from build123d import *

# Parameters (mm, degrees)
F0_W     = 101.6
F0_H     = 76.2
F1_DEPTH = 76.2
F3_DEPTH = 76.201
F5_DEPTH = 50.8


with BuildPart() as f1:
    # F0 (on Front) → F1 (new body)
    with BuildSketch(Plane.XZ):
        with Locations((21.473836, 21.002229)):
            Rectangle(F0_W, F0_H)
    extrude(amount=F1_DEPTH)

    # F2 (on face) → F3 (cut, through all)
    with BuildSketch(Plane.XY.offset(59.102229)):
        with BuildLine():
            Line((72.273836, -63.5), (72.273836, -12.7))
            ThreePointArc((72.273836, -12.7), (46.873836, -38.1), (72.273836, -63.5))
        make_face()
    extrude(amount=-F3_DEPTH, mode=Mode.SUBTRACT)

    # F4 (on face) → F5 (cut)
    with BuildSketch(Plane(origin=(-29.326164, 0, 0), x_dir=(0, -1, 0), z_dir=(-1, 0, 0))):
        with BuildLine():
            Line((76.2, 59.102229), (25.4, 59.102229))
            ThreePointArc((25.4, 59.102229), (40.278976, 23.181204), (76.2, 8.302229))
            Line((76.2, 8.302229), (76.2, 59.102229))
        make_face()
    extrude(amount=-F5_DEPTH, mode=Mode.SUBTRACT)


solid = f1.part
Work out the finished part from the listing and answer in its coordinate system (mm). A direction names the side the tool comes from. Round coordinates to 2 decimals unless told otherwise and drop trailing zeros. Write each loop counter-clockwise with the first axis right and the second up, starting at its lowest first coordinate (ties: lowest second). Pieces come first, ordered by that corner, then holes. Notation, with made-up numbers: M 57.25,-17.75 L 68.25,-17.75 A32 cw 68.25,12.25 Z; hole C 40.5,29 d10. An arc over 180 degrees is marked long. Use a Markdown table: item, result.
1) Consider line 1 (Y direction, x = 53, z = 53); line 2 (X direction, y = -41.5, z = 54.5); line 3 (X direction, y = -31, z = 43). Determine where each line is inside the solid, lowest interval first. Write a range as [from, to].
Taken from the geometry:
| item | result |
|---|---|
| line 1 | y = [-76.2, -54.64], [-21.56, 0] |
| line 2 | x = [21.47, 47.1] |
| line 3 | x = [21.47, 47.89] |
2) Which of the six approach directions +Z, -Z, +X, -X, +Y, -Y give full straight-line access (tool end or side, diameter ignored) to faces 4 (the face through (72.274, -70, 20)), 5 (the face through (-4.282, -39.886, 23.578))?
Taken from the geometry:
| item | result |
|---|---|
| face 4 | +Z, -Z, +X, +Y, -Y |
| face 5 | +Z, -X, -Y |
3) Determine the mould class of faces 1 (the face through (72.274, -6, 20)), 2 (the face through (46.88, -37.54, 21.54)), 3 (the face through (21, 0, 22)) for opening direction Y: pulls with the +Y half, pulls with the -Y half, needs draft (parallel to the pull), parting line crosses it, or undercut.
Taken from the geometry:
| item | result |
|---|---|
| face 1 | needs draft |
| face 2 | undercut |
| face 3 | pulls with the +Y half |
4) The part is cut by section B-B on z = 17. Give the vertices of the cut face in (x, y).
Taken from the geometry:
| item | result |
|---|---|
| outline | M -29.33,-47.77 L 21.47,-47.77 L 21.47,-76.2 L 72.27,-76.2 L 72.27,-63.5 A25.4 cw 72.27,-12.7 L 72.27,0 L -29.33,0 Z |
5) The part is cut by section D-D on y = -38.1. Give the vertices of the cut face in (x, z).
Taken from the geometry:
| item | result |
|---|---|
| outline | M -29.33,-17.1 L 46.87,-17.1 L 46.87,59.1 L 21.47,59.1 L 21.47,25.5 L -29.33,25.5 Z |
6) The part is cut by section A-A on x = 16. Give the vertices of the cut face in (y, z).
Taken from the geometry:
| item | result |
|---|---|
| outline | M -76.2,-17.1 L 0,-17.1 L 0,59.1 L -25.4,59.1 A50.8 cw -76.2,8.3 Z |
7) Flat-ended cylindrical pins translate along their axes: pin 1 (1.5 mm diameter, centred on x = 14, z = 23, fed in from -Y) (3 decimals); pin 2 (1 mm diameter, centred on y = -40, z = 36.5, fed in from +X). Find the tip coordinate at first contact, or state that the pin passes through.
Taken from the geometry:
| item | result |
|---|---|
| pin 1 | stops at y = -41.235 |
| pin 2 | stops at x = 46.99 |
8) The part is cut by section C-C on x = 55. Give the vertices of the cut face in (y, z), plus the area to 3 significant figures.
Taken from the geometry:
| item | result |
|---|---|
| outline | M -76.2,-17.1 L -56.72,-17.1 L -56.72,59.1 L -76.2,59.1 Z; M -19.48,-17.1 L 0,-17.1 L 0,59.1 L -19.48,59.1 Z |
| area | 2,970 mm2 |
